Source: CAD feature listing. Evaluate the final solid. Frame: model axes, mm. Face numbers are marked on the shaded views. A direction names the side the tool comes from. Give positions to 0.01 mm unless a question says otherwise; leave off trailing zeros. Loops run counter-clockwise (first coordinate to the right, second up) from the corner with the lowest first, then second, coordinate; pieces in that order, holes last.
```python
from build123d import *

# Parameters (mm, degrees)
SALIENTE_EXTRUIR1_DEPTH      = 20
TALADRO_DE_MARGEN_PARA_M31_D = 3.6
REDONDEO1_R                  = 1
CORTAR_EXTRUIR1_REACH        = 40.303


with BuildPart() as part:
    # Croquis1 → Saliente-Extruir1 (new body)
    with BuildSketch(Plane.XY):
        with BuildLine():
            Line((-12.55, 0), (-21.55, 0))
            Line((-21.55, 0), (-21.55, 2))
            Line((-21.55, 2), (-14.55, 2))
            Line((-14.55, 2), (-14.55, 12))
            ThreePointArc((-14.55, 12), (0, 26.55), (14.55, 12))
            Line((14.55, 12), (14.55, 2))
            Line((14.55, 2), (21.55, 2))
            Line((21.55, 2), (21.55, 0))
            Line((21.55, 0), (12.55, 0))
            Line((12.55, 0), (12.55, 12))
            ThreePointArc((12.55, 12), (0, 24.55), (-12.55, 12))
            Line((-12.55, 12), (-12.55, 0))
        make_face()
    extrude(amount=SALIENTE_EXTRUIR1_DEPTH)

    # Taladro de margen para M31 (through all)
    with Locations(Plane(origin=(0, 2, 0), x_dir=(1, 0, 0), z_dir=(0, 1, 0))):
        with Locations((18.05, -10), (-18.05, -10)):
            Hole(TALADRO_DE_MARGEN_PARA_M31_D / 2)

    # Redondeo1
    redondeo1_edges = [part.edges().sort_by_distance(p)[0] for p in [
        (14.55, 2, 10),
        (-14.55, 2, 10),
    ]]
    fillet(redondeo1_edges, radius=REDONDEO1_R)

    # Croquis4 → Cortar-Extruir1 (cut, up to next)
    with BuildSketch(Plane(origin=(0, 2, 0), x_dir=(1, 0, 0), z_dir=(0, 1, 0)), mode=Mode.PRIVATE) as cortar_extruir1_sk1:
        with BuildLine():
            Line((-18.815101364, -8.370699567), (-18.05, -8.011416474))
            Line((-18.05, -8.011416474), (-17.284898636, -8.370699567))
            ThreePointArc((-17.284898636, -8.370699567), (-18.05, -8.2), (-18.815101364, -8.370699567))
        make_face()
    cortar_extruir1_tool1 = extrude(cortar_extruir1_sk1.sketch, amount=-CORTAR_EXTRUIR1_REACH, mode=Mode.PRIVATE) & part.part
    cortar_extruir1 = cortar_extruir1_tool1.solids().sort_by_distance((-18.05, 2, 8.160025))[0]
    add(cortar_extruir1, mode=Mode.SUBTRACT)

    # Simetría1: Cortar-Extruir1 across plane
    add(cortar_extruir1.mirror(Plane(origin=(0, 0, 0), x_dir=(0, 0, 1), z_dir=(1, 0, 0))), mode=Mode.SUBTRACT)


solid = part.part
```
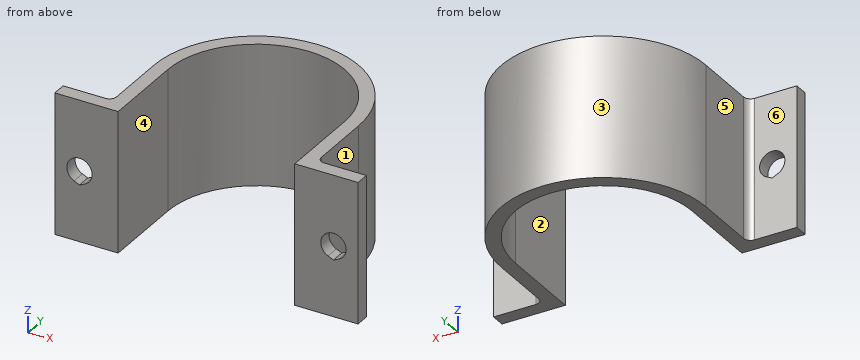
(1) Section D-D, the plane y = 12.5. Return the cut outline in (x, z).
A:
outline: (-14.54, 0) - (-12.54, 0) - (-12.54, 20) - (-14.54, 20) - close; (12.54, 0) - (14.54, 0) - (14.54, 20) - (12.54, 20) - close
(2) Section B-B, the plane y = 7.75. Return the cut outline in (x, z), then the cut area to 3 significant figures.
A:
outline: (-14.55, 0) - (-12.55, 0) - (-12.55, 20) - (-14.55, 20) - close; (12.55, 0) - (14.55, 0) - (14.55, 20) - (12.55, 20) - close
area: 80.0 mm2
(3) Section A-A, the plane z = 10. Return the cut outline in (x, y).
A:
outline: (-21.55, 0) - (-19.85, 0) - (-19.85, 2) - (-21.55, 2) - close; (-16.25, 0) - (-12.55, 0) - (-12.55, 12) arc R12.55 cw to (12.55, 12) - (12.55, 0) - (16.25, 0) - (16.25, 2) - (15.55, 2) arc R1 cw to (14.55, 3) - (14.55, 12) arc R14.55 ccw to (-14.55, 12) - (-14.55, 3) arc R1 cw to (-15.55, 2) - (-16.25, 2) - close; (19.85, 0) - (21.55, 0) - (21.55, 2) - (19.85, 2) - close
(4) Reachability of the marked faces 1, 2 and 3 from +Z, -Z, +X, -X, +Y, -Y: full face, straight path, thin tool, end or side. Return the list, or none.
A:
face 1: +Z, -Z, +X, +Y
face 2: +Z, -Z, -Y
face 3: +Z, -Z, +Y
(5) Ray query, line 1 along X through (y, z) = (0.85, 10); line 2 along Z through (x, y) = (-18.05, 0.85); line 3 along X through (y, z) = (7.75, 15.5). Return the intervals inside material, ascending.
A:
line 1: x = -21.55 to -19.85, -16.25 to -12.55, 12.55 to 16.25, 19.85 to 21.55
line 2: z = 0 to 8.01, 11.8 to 20
line 3: x = -14.55 to -12.55, 12.55 to 14.55
(6) Mould query, pull axis X, two halves, no side actions, for the marked faces 4, 5 and 6. Classes: pulls with the +X half, pulls with the -X half, needs draft (parallel to the pull), parting line crosses it, or undercut.
A:
face 4: undercut
face 5: pulls with the -X half
face 6: needs draft
(7) First-contact query: pin 1 (5 mm diameter, centred on x = -11.5, z = 12.5, fed in from +Y); pin 2 (1.5 mm diameter, centred on y = 12, z = 4.5, fed in from -X); pin 3 (9.5 mm diameter, centred on y = 7.5, z = 6.5, fed in from +X); pin 4 (3 mm diameter, centred on x = 18.05, z = 10, fed in from +Y). Flat tips, straight axial feed; report the tip coordinate or a pass-through.
A:
pin 1: stops at y = 23.43
pin 2: stops at x = -14.55
pin 3: stops at x = 14.58
pin 4: passes through
(8) Section C-C, the plane z = 14.5. Return the cut outline in (x, y), then the cut area to 3 significant figures.
A:
outline: (-21.55, 0) - (-12.55, 0) - (-12.55, 12) arc R12.55 cw to (12.55, 12) - (12.55, 0) - (21.55, 0) - (21.55, 2) - (15.55, 2) arc R1 cw to (14.55, 3) - (14.55, 12) arc R14.55 ccw to (-14.55, 12) - (-14.55, 3) arc R1 cw to (-15.55, 2) - (-21.55, 2) - close
area: 162 mm2
